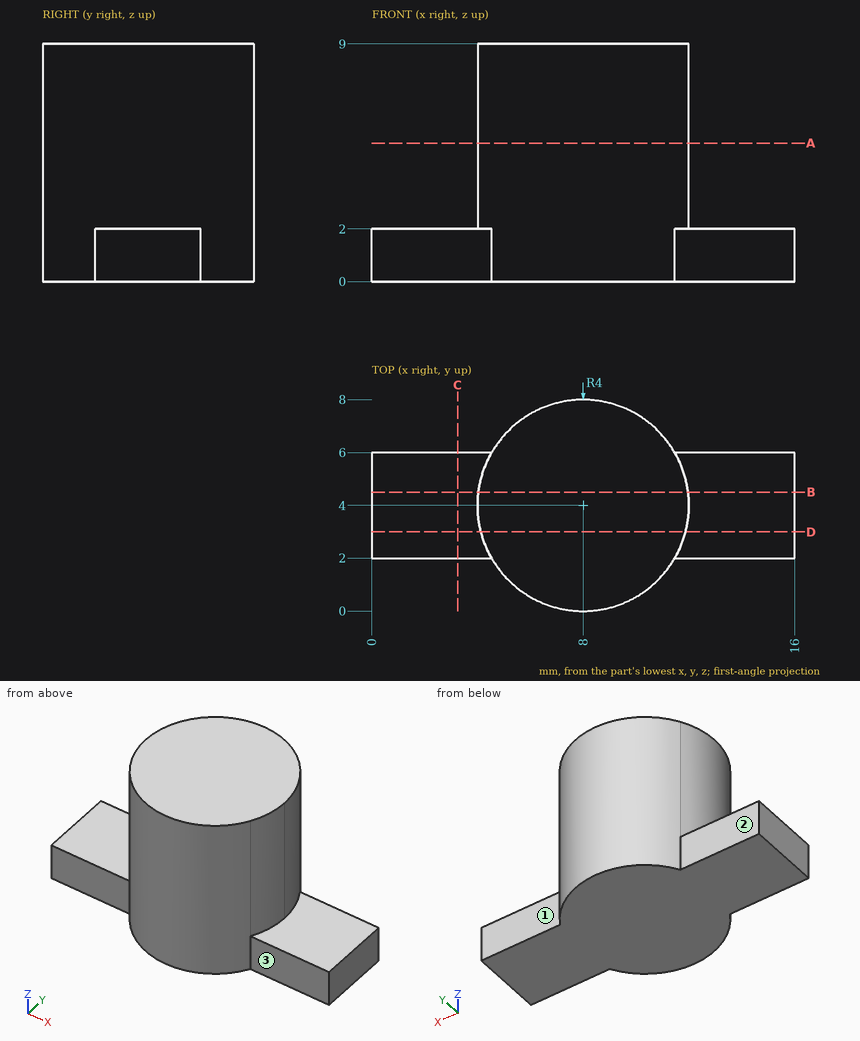
Here's the drawing with two shaded views (mm, measured from the low corner). I have some questions. A direction names the side the tool comes from. Coordinates: 2 decimals unless noted, no trailing zeros. Order: outer loops, then holes, each group sorted by start corner. A loop starts at its lowest first (then second) coordinate and runs counter-clockwise, first axis right, second up. Notation, with made-up numbers: (22, 10) - (72, 10) arc R11 ccw to (72, 26) - close; hole circle Ø4 at (-31, 85). An arc over 180 degrees is marked (long way). Use CSV: the item, a comma, the result in double quotes. Start each with the question number.
1. I'm going to push flat-ended pins straight in: pin 1 (2 mm diameter, centred on x = 14.5, z = 1.5, fed in from -Y); pin 2 (0.6 mm diameter, centred on x = 14.5, z = 0.5, fed in from +Y); pin 3 (4 mm diameter, centred on y = 1, z = 6, fed in from +X). Where does each tip first touch, or does it pass through?
2. Suppose I cut it at A-A on z = 5.25. List the corners of the cut face in (x, y) for me, then the cut area to 3 significant figures.
3. For the marked faces 1, 2 and 3, which set-ups out of +Z, -Z, +X, -X, +Y, -Y let a thin tool reach every point of the face, with its end or its side?
4. Suppose I cut it at C-C on x = 3.25. List the corners of the cut face in (y, z) for me.
5. Suppose I cut it at D-D on y = 3. List the corners of the cut face in (x, z) for me.
6. Suppose I cut it at B-B on y = 4.5. List the corners of the cut face in (x, z) for me, then the cut area to 3 significant figures.
7. Please list where these lines run through material, in increasing order: line 1 (Y direction, x = 3.75, z = 0.75); line 2 (Z direction, x = 1.5, y = 4); line 3 (Y direction, x = 7.5, z = 1). Write a range as from..to.
Output:
1,pin 1,"stops at y = 2"
1,pin 2,"stops at y = 6"
1,pin 3,"stops at x = 11.87"
2,outline,"circle Ø8 at (8, 4)"
2,area,"50.3 mm2"
3,face 1,"+Z, -Z, +X, +Y"
3,face 2,"+Z, -Z, -X, +Y"
3,face 3,"+Z, -Z, +X, -Y"
4,outline,"(2, 0) - (6, 0) - (6, 2) - (2, 2) - close"
5,outline,"(0, 0) - (16, 0) - (16, 2) - (11.87, 2) - (11.87, 9) - (4.13, 9) - (4.13, 2) - (0, 2) - close"
6,outline,"(0, 0) - (16, 0) - (16, 2) - (11.97, 2) - (11.97, 9) - (4.03, 9) - (4.03, 2) - (0, 2) - close"
6,area,"87.6 mm2"
7,line 1,"y = 2..6"
7,line 2,"z = 0..2"
7,line 3,"y = 0.03..7.97"
